Design review of the part built by this model. Coordinates are the model's own, in mm. A direction names the side the tool comes from. Give positions to 0.01 mm unless a question says otherwise; leave off trailing zeros. Order: outer loops, then holes, each group sorted by start corner. A loop starts at its lowest first (then second) coordinate and runs counter-clockwise, first axis right, second up. Notation, with made-up numbers: (0, 27.5) -> (21, 27.5) arc R20 cw to (21, 64.5) -> close; hole circle Ø8 at (9.5, 45.5). An arc over 180 degrees is marked (long way). Return JSON: item names as keys, results as strings.
```python
from build123d import *

# Parameters (mm, degrees)
SKETCH10_R         = 6
CUT_EXTRUDE2_DEPTH = 184.098334236
CUT_EXTRUDE4_DEPTH = 184.098334236
CUT_EXTRUDE4_DRAFT = -0.57


with BuildPart() as part:
    # Sketch2 → Revolve1 (revolve)
    with BuildSketch(Plane(origin=(0, 0, 0), x_dir=(1, 0, 0), z_dir=(0, 1, 0))):
        with BuildLine():
            Line((0, 22.5), (0, 5))
            ThreePointArc((0, 5), (1.464466094, 1.464466094), (5, 0))
            Line((5, 0), (45, 0))
            ThreePointArc((45, 0), (48.535533906, -1.464466094), (50, -5))
            Line((50, -5), (50, -45))
            ThreePointArc((50, -45), (51.464466094, -48.535533906), (55, -50))
            Line((55, -50), (70, -50))
            Line((70, -50), (70, 22.5))
            Line((70, 22.5), (0, 22.5))
        make_face()
    revolve(axis=Axis((0, 0, -45), (1, 0, 0)))

    # Sketch10 → Cut-Extrude2 (cut, through all)
    with BuildSketch(Plane(origin=(70, 0, 0), x_dir=(0, 0, -1), z_dir=(1, 0, 0))):
        with Locations((45, -70)):
            Circle(SKETCH10_R)
        with Locations((-25, 0)):
            Circle(SKETCH10_R)
        with Locations((45, 70)):
            Circle(SKETCH10_R)
        with Locations((115, 0)):
            Circle(SKETCH10_R)
    extrude(amount=-CUT_EXTRUDE2_DEPTH, mode=Mode.SUBTRACT)


with BuildPart() as cut_extrude4_tool:
    # Sketch11 → Cut-Extrude4 (with draft: the straight prism first)
    with BuildSketch(Plane(origin=(70, 0, 0), x_dir=(0, 0, -1), z_dir=(1, 0, 0))):
        Polygon((38, 25.4), (38, 21.38340478), (38, 21.284496071), (52, 21.38340478), (52, 25.4), (45, 25.4), align=None)
    extrude(amount=-CUT_EXTRUDE4_DEPTH)
    # Cut-Extrude4: the draft: its side faces are tilted about the plane it starts from
    cut_extrude4_sides = [cut_extrude4_tool.faces().sort_by_distance(p)[0] for p in [
        (-22.049167118, 23.342248035, -38),
        (-22.049167118, 23.39170239, -52),
        (-22.049167118, 21.333950426, -45),
        (-22.049167118, 25.4, -45),
    ]]
    draft(cut_extrude4_sides, Plane(origin=(70, 0, 0), x_dir=(0, 0, -1), z_dir=(1, 0, 0)), CUT_EXTRUDE4_DRAFT)


with BuildPart() as part_1:
    add(part.part)

    # Cut-Extrude4: cut by cut_extrude4_tool
    add(cut_extrude4_tool.part, mode=Mode.SUBTRACT)


solid = part_1.part
```
Item 1: Add section A-A (y = 0). Give the boundary of the cut face in (x, z).
Result set:
{"outline": "(0, -85) arc R5 ccw to (5, -90) -> (45, -90) arc R5 cw to (50, -95) -> (50, -109) -> (70, -109) -> (70, -67.5) -> (0, -67.5) -> close; (0, -22.5) -> (70, -22.5) -> (70, 19) -> (50, 19) -> (50, 5) arc R5 cw to (45, 0) -> (5, 0) arc R5 ccw to (0, -5) -> close; (50, -135) arc R5 ccw to (55, -140) -> (70, -140) -> (70, -121) -> (50, -121) -> close; (50, 31) -> (70, 31) -> (70, 50) -> (55, 50) arc R5 ccw to (50, 45) -> close"}
Item 2: Add section B-B (z = -45). Give the boundary of the cut face in (x, y).
Result set:
{"outline": "(0, -40) arc R5 ccw to (5, -45) -> (45, -45) arc R5 cw to (50, -50) -> (50, -64) -> (70, -64) -> (70, -22.5) -> (0, -22.5) -> close; (0, 24.7) -> (70, 25.4) -> (70, 64) -> (50, 64) -> (50, 50) arc R5 cw to (45, 45) -> (5, 45) arc R5 ccw to (0, 40) -> close; (50, -90) arc R5 ccw to (55, -95) -> (70, -95) -> (70, -76) -> (50, -76) -> close; (50, 76) -> (70, 76) -> (70, 95) -> (55, 95) arc R5 ccw to (50, 90) -> close"}
Item 3: Wall thickness on L1, parallel to Y at x = 65, z = -45; L2, parallel to Z at x = 21, y = 0; L3, parallel to Y at x = 60.5, z = -45: over which ranges is each line inside the solid? List them lowest first. Write a range as [from, to].
Result set:
{"L1": "y = [-95, -76], [-64, -22.5], [25.35, 64], [76, 95]", "L2": "z = [-90, -67.5], [-22.5, 0]", "L3": "y = [-95, -76], [-64, -22.5], [25.31, 64], [76, 95]"}
Item 4: For pin 1 (7 mm diameter, centred on y = 0, z = 25, fed in from +X); pin 2 (12 mm diameter, centred on x = 61, z = -12, fed in from -Y); pin 3 (14 mm diameter, centred on y = 70, z = -45, fed in from +X); pin 4 (8 mm diameter, centred on x = 16, z = -51, fed in from -Y), all flat-tipped, find the tip position at first contact; note any pin that passes through.
Result set:
{"pin 1": "passes through", "pin 2": "stops at y = -91.08", "pin 3": "stops at x = 70", "pin 4": "stops at y = -44.96"}
Item 5: Machinability: for faces 1 (the face through (50, 39, -84)), 2 (the face through (0, 17, -62)), which of the approach directions +Z, -Z, +X, -X, +Y, -Y give a long, thin tool a straight path to every point of the face, cutting with its end or side? Answer none if there is none.
Result set:
{"face 1": "-X", "face 2": "+Z, -Z, -X, +Y, -Y"}
Item 6: Mouldability with a two-part tool opening along Y and no side actions: class faces 3 (the face through (70, 20, -25)), 4 (the face through (34.51, -22.487, -44.234)), 5 (the face through (60.14, -65.94, -40.58)), 6 (the face through (25.28, -1.979, -89.956)) as released by +Y, released by -Y, zero draft, split by the parting line, or undercut.
Result set:
{"face 3": "zero draft", "face 4": "undercut", "face 5": "undercut", "face 6": "split by the parting line"}
Item 7: Add section C-C (x = 37.5). Give the boundary of the cut face in (y, z), plus the area to 3 significant figures.
Result set:
{"outline": "circle Ø90 at (0, -45); hole (21.61, -38.75) arc R22.5 ccw (long way) to (21.7, -50.95) -> (21.7, -51.68) -> (25.08, -51.68) -> (25.08, -38.32) -> (21.61, -38.32) -> close", "area": "4,730 mm^2"}
